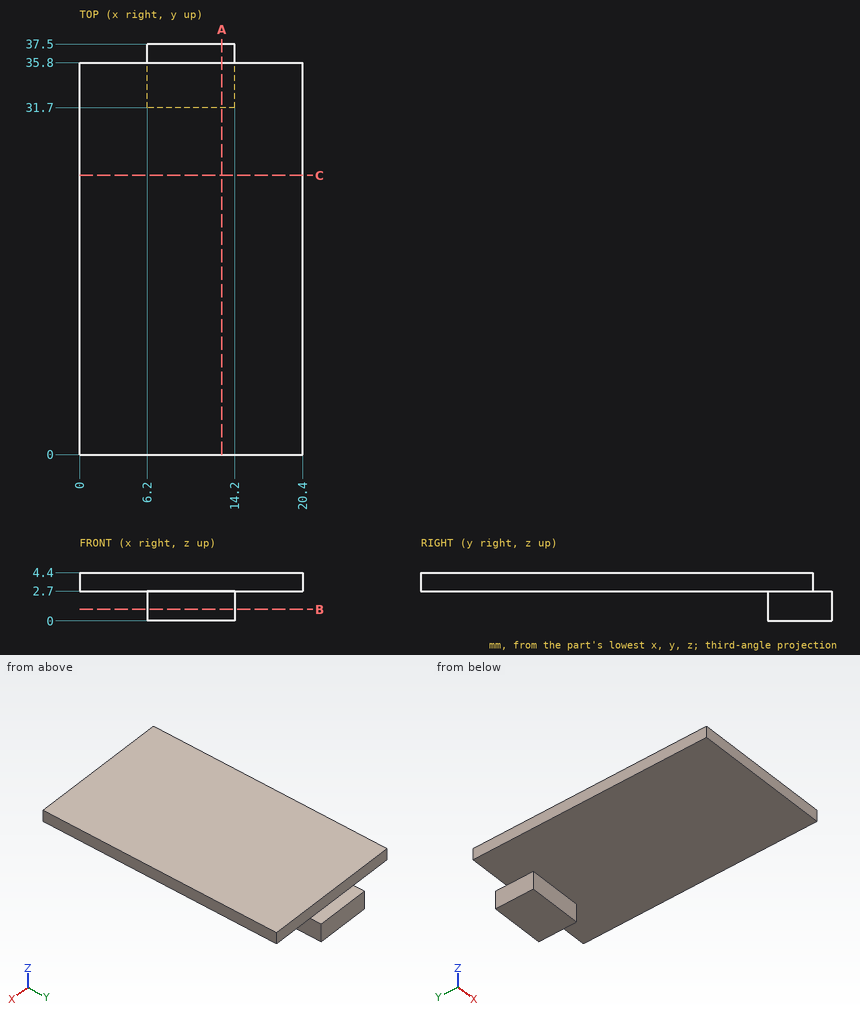
Source: three-view drawing plus pictorial views. Frame: mm from the lowest corner of the part. Give positions to 0.01 mm unless a question says otherwise; leave off trailing zeros. Write each loop counter-clockwise with the first axis right and the second up, starting at its lowest first coordinate (ties: lowest second). Pieces come first, ordered by that corner, then holes.
(1) Cut plane B-B, the plane z = 1.05. Return loops of the section in (x, y).
(2) Cut plane A-A, the plane x = 13. Return loops of the section in (y, z).
(3) Cut plane C-C, the plane y = 25.5. Return loops of the section in (x, z).
(4) Ray query, line 1 (Y direction, x = 13.5, z = 1.1); line 2 (Y direction, x = 3.5, z = 3.8); line 3 (Z direction, x = 18.25, y = 17.5). Return the intervals inside material, ascending.
(5) First-contact query: P1, Ø0.8, axis at y = 35, z = 1.5, coming from the +X side; P2, Ø1.4, axis at x = 9, z = 1.5, coming from the -Y side; P3, Ø0.5, axis at x = 10.5, y = 37, coming from the +Z side. Flat tips, straight axial feed; report the tip coordinate or a pass-through.
Values follow:
1. outline: (6.2, 31.7) - (14.2, 31.7) - (14.2, 37.5) - (6.2, 37.5) - close
2. outline: (0, 2.7) - (31.7, 2.7) - (31.7, 0) - (37.5, 0) - (37.5, 2.7) - (35.8, 2.7) - (35.8, 4.4) - (0, 4.4) - close
3. outline: (0, 2.7) - (20.4, 2.7) - (20.4, 4.4) - (0, 4.4) - close
4. line 1: y = 31.7 to 37.5
4. line 2: y = 0 to 35.8
4. line 3: z = 2.7 to 4.4
5. P1: stops at x = 14.2
5. P2: stops at y = 31.7
5. P3: stops at z = 2.7
